Design review of the part built by this model. Coordinates are the model's own, in mm. A direction names the side the tool comes from. Coordinates: 2 decimals unless noted, no trailing zeros. Loops run counter-clockwise (first coordinate to the right, second up) from the corner with the lowest first, then second, coordinate; pieces in that order, holes last. Notation, with made-up numbers: (-33, 55) - (-25, 55) arc R27 cw to (-25, 73) - close; hole circle Ø4 at (40.25, -18.5). An arc over 180 degrees is marked (long way). One line per question, with ' | ' between items.
from build123d import *

# Parameters (mm, degrees)
F0_R     = 1.6
F0_W     = 30
F0_H     = 4
F0_W_2   = 4
F0_H_2   = 30
F1_DEPTH = 4


with BuildPart() as f1:
    # F0 (on Right) → F1 (new body)
    with BuildSketch(Plane.YZ):
        with BuildLine():
            Line((-119.978741, -65.165301), (-119.978741, -61.165301))
            Line((-119.978741, -61.165301), (-99.978741, -61.165301))
            Line((-99.978741, -61.165301), (-99.978741, -65.165301))
            Line((-99.978741, -65.165301), (-79.978741, -65.165301))
            Line((-79.978741, -65.165301), (-79.978741, -61.165301))
            Line((-79.978741, -61.165301), (-59.978741, -61.165301))
            Line((-59.978741, -61.165301), (-59.978741, -65.165301))
            Line((-59.978741, -65.165301), (-39.978741, -65.165301))
            Line((-39.978741, -65.165301), (-39.978741, -61.165301))
            Line((-39.978741, -61.165301), (-19.978741, -61.165301))
            Line((-19.978741, -61.165301), (-19.978741, -65.165301))
            Line((-19.978741, -65.165301), (0.021259, -65.165301))
            Line((0.021259, -65.165301), (0.021259, -61.165301))
            Line((0.021259, -61.165301), (20.021259, -61.165301))
            Line((20.021259, -61.165301), (20.021259, -65.165301))
            Line((20.021259, -65.165301), (20.021259, -75.818613))
            ThreePointArc((20.021259, -75.818613), (25.021259, -78.165301), (30.021259, -75.818613))
            Line((30.021259, -75.818613), (30.021259, -65.165301))
            Line((30.021259, -65.165301), (30.021259, -61.165301))
            Line((30.021259, -61.165301), (30.021259, 84.834699))
            Line((30.021259, 84.834699), (-129.978741, 84.834699))
            Line((-129.978741, 84.834699), (-133.978741, 84.834699))
            Line((-133.978741, 84.834699), (-133.978741, 64.834699))
            Line((-133.978741, 64.834699), (-129.978741, 64.834699))
            Line((-129.978741, 64.834699), (-129.978741, 44.834699))
            Line((-129.978741, 44.834699), (-133.978741, 44.834699))
            Line((-133.978741, 44.834699), (-133.978741, 24.834699))
            Line((-133.978741, 24.834699), (-129.978741, 24.834699))
            Line((-129.978741, 24.834699), (-129.978741, 4.834699))
            Line((-129.978741, 4.834699), (-133.978741, 4.834699))
            Line((-133.978741, 4.834699), (-133.978741, -15.165301))
            Line((-133.978741, -15.165301), (-129.978741, -15.165301))
            Line((-129.978741, -15.165301), (-129.978741, -35.165301))
            Line((-129.978741, -35.165301), (-133.978741, -35.165301))
            Line((-133.978741, -35.165301), (-133.978741, -55.165301))
            Line((-133.978741, -55.165301), (-129.978741, -55.165301))
            Line((-129.978741, -55.165301), (-129.978741, -65.165301))
            Line((-129.978741, -65.165301), (-119.978741, -65.165301))
        make_face()
        with Locations((-61.353443, -45.165301)):
            Circle(F0_R, mode=Mode.SUBTRACT)
        with Locations((-104.978741, -10.165301)):
            Rectangle(F0_W, F0_H, mode=Mode.SUBTRACT)
        with Locations((-77.978741, -36.165301)):
            Rectangle(F0_W_2, F0_H_2, mode=Mode.SUBTRACT)
        with Locations((-61.353443, -25.165301)):
            Circle(F0_R, mode=Mode.SUBTRACT)
        with Locations((-61.353443, -5.165301)):
            Circle(F0_R, mode=Mode.SUBTRACT)
        with Locations((-41.353443, -45.165301)):
            Circle(F0_R, mode=Mode.SUBTRACT)
        with Locations((-21.353443, -45.165301)):
            Circle(F0_R, mode=Mode.SUBTRACT)
        with Locations((-1.353443, -45.165301)):
            Circle(F0_R, mode=Mode.SUBTRACT)
        with Locations((18.646557, -45.165301)):
            Circle(F0_R, mode=Mode.SUBTRACT)
        with Locations((-41.353443, -25.165301)):
            Circle(F0_R, mode=Mode.SUBTRACT)
        with Locations((-21.353443, -25.165301)):
            Circle(F0_R, mode=Mode.SUBTRACT)
        with Locations((-41.353443, -5.165301)):
            Circle(F0_R, mode=Mode.SUBTRACT)
        with Locations((-21.353443, -5.165301)):
            Circle(F0_R, mode=Mode.SUBTRACT)
        with Locations((-1.353443, -25.165301)):
            Circle(F0_R, mode=Mode.SUBTRACT)
        with Locations((18.646557, -25.165301)):
            Circle(F0_R, mode=Mode.SUBTRACT)
        with Locations((-1.353443, -5.165301)):
            Circle(F0_R, mode=Mode.SUBTRACT)
        with Locations((18.646557, -5.165301)):
            Circle(F0_R, mode=Mode.SUBTRACT)
        with Locations((-61.353443, 14.834699)):
            Circle(F0_R, mode=Mode.SUBTRACT)
        with Locations((-61.353443, 34.834699)):
            Circle(F0_R, mode=Mode.SUBTRACT)
        with Locations((-61.353443, 54.834699)):
            Circle(F0_R, mode=Mode.SUBTRACT)
        with Locations((-61.353443, 74.834699)):
            Circle(F0_R, mode=Mode.SUBTRACT)
        with Locations((-41.353443, 14.834699)):
            Circle(F0_R, mode=Mode.SUBTRACT)
        with Locations((-21.353443, 14.834699)):
            Circle(F0_R, mode=Mode.SUBTRACT)
        with Locations((-41.353443, 34.834699)):
            Circle(F0_R, mode=Mode.SUBTRACT)
        with Locations((-21.353443, 34.834699)):
            Circle(F0_R, mode=Mode.SUBTRACT)
        with Locations((-1.353443, 14.834699)):
            Circle(F0_R, mode=Mode.SUBTRACT)
        with Locations((18.646557, 14.834699)):
            Circle(F0_R, mode=Mode.SUBTRACT)
        with Locations((-1.353443, 34.834699)):
            Circle(F0_R, mode=Mode.SUBTRACT)
        with Locations((18.646557, 34.834699)):
            Circle(F0_R, mode=Mode.SUBTRACT)
        with Locations((-41.353443, 54.834699)):
            Circle(F0_R, mode=Mode.SUBTRACT)
        with Locations((-21.353443, 54.834699)):
            Circle(F0_R, mode=Mode.SUBTRACT)
        with Locations((-41.353443, 74.834699)):
            Circle(F0_R, mode=Mode.SUBTRACT)
        with Locations((-21.353443, 74.834699)):
            Circle(F0_R, mode=Mode.SUBTRACT)
        with Locations((-1.353443, 54.834699)):
            Circle(F0_R, mode=Mode.SUBTRACT)
        with Locations((18.646557, 54.834699)):
            Circle(F0_R, mode=Mode.SUBTRACT)
        with Locations((-1.353443, 74.834699)):
            Circle(F0_R, mode=Mode.SUBTRACT)
        with Locations((18.646557, 74.834699)):
            Circle(F0_R, mode=Mode.SUBTRACT)
    extrude(amount=F1_DEPTH)


solid = f1.part
Q1. Tool access review of faces 5 (the flat face through (0, -53, 4)), 6 (the flat face through (2, -70, -61.165)), 7 (the flat face through (2, -132, 64.835)), 8 (the flat face through (2, -119.979, -10)), 9 (the flat face through (2, -50, -65.165)): name each direction out of +Z, -Z, +X, -X, +Y, -Y from which nothing blocks a thin tool from reaching the whole face with its end or side.
Returned:
face 5: +Z, -Z, -X, +Y, -Y | face 6: -Z, +X, -X | face 7: +X, -X, -Y | face 8: +X, -X | face 9: -Z, +X, -X, -Y
Q2. To check wall thickness, follow line 1 along Y through (x, z) = (3.55, -63); line 2 along Y through (x, z) = (1.85, 15); line 3 along Y through (x, z) = (3.4, -33). State the ranges of each line that lie inside material, in increasing order.
Returned:
line 1: y = -129.98 to -119.98, -99.98 to -79.98, -59.98 to -39.98, -19.98 to 0.02, 20.02 to 30.02 | line 2: y = -129.98 to -62.94, -59.76 to -42.94, -39.76 to -22.94, -19.76 to -2.94, 0.24 to 17.06, 20.24 to 30.02 | line 3: y = -129.98 to -79.98, -75.98 to 30.02
Q3. Take a section at B-B (y = -55). Give the boundary of the cut face in (x, z), plus the area to 3 significant figures.
Returned:
outline: (0, -65.17) - (4, -65.17) - (4, 84.83) - (0, 84.83) - close | area: 600 mm²
Q4. Take a section at C-C (z = 20). Give the boundary of the cut face in (x, y).
Returned:
outline: (0, -129.98) - (4, -129.98) - (4, 30.02) - (0, 30.02) - close
Q5. For pin 1 (3 mm diameter, centred on y = -21.35, z = 34.83, fed in from -X); pin 2 (1.2 mm diameter, centred on x = 2, y = -26.5, fed in from -Z); pin 3 (1.2 mm diameter, centred on x = 2.5, z = -62, fed in from -Y); pin 4 (2 mm diameter, centred on x = 2, y = -132.5, fed in from -Z), all flat-tipped, find the tip position at first contact; note any pin that passes through.
Returned:
pin 1: passes through | pin 2: stops at z = -61.17 | pin 3: stops at y = -129.98 | pin 4: stops at z = -55.17
Q6. Take a section at A-A (y = -113). Give the boundary of the cut face in (x, z).
Returned:
outline: (0, -61.17) - (4, -61.17) - (4, -12.17) - (0, -12.17) - close; (0, -8.17) - (4, -8.17) - (4, 84.83) - (0, 84.83) - close
Q7. Draft analysis for pull direction Y (two halves, no side actions). For faces 1 (the flat face through (2, -129.979, -60)), 2 (the cylindrical face through (1.972, 24.941, -78.165)), 3 (the flat face through (2, -30, -61.165)), 4 (the flat face through (2, -125, -65.165)), state which applies: +Y half, -Y half, draft (parallel to the pull), parting line (faces both ways), or undercut.
Returned:
face 1: -Y half | face 2: parting line | face 3: undercut | face 4: draft
Q8. Take a section at D-D (x = 2.45). State how many separate pieces and enclosed holes the cut face has, plus the area to 3 significant figures.
Returned:
separate pieces: 1 | enclosed holes: 37 | area: 23,600 mm²
